CAD build for the part. Positions are in the model's coordinates, mm. Round coordinates to 2 decimals unless told otherwise and drop trailing zeros. Loops run counter-clockwise (first coordinate to the right, second up) from the corner with the lowest first, then second, coordinate; pieces in that order, holes last. Notation, with made-up numbers: (-20, 16.5) - (22, 16.5) arc R24 ccw to (22, 47.5) - close; hole circle Ø3 at (-16, 88). An arc over 180 degrees is marked (long way). One line per question, with ' | ' between items.
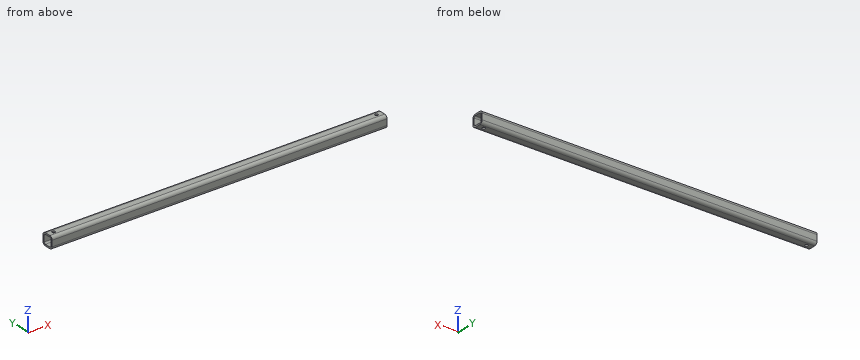
```python
from build123d import *

# Parameters (mm, degrees)
STRUCTURAL_MEMBER1_DEPTH = 1422.4
SKETCH12_R               = 6.35
CUT_EXTRUDE1_DEPTH       = 744.764894646


with BuildPart() as part:
    # Sketch11 → Structural Member1 (new body)
    with BuildSketch(Plane.YZ.offset(-741.593162393)):
        with BuildLine():
            Line((-12.7, -25.4), (12.7, -25.4))
            ThreePointArc((12.7, -25.4), (21.680256121, -21.680256121), (25.4, -12.7))
            Line((25.4, -12.7), (25.4, 12.7))
            ThreePointArc((25.4, 12.7), (21.680256121, 21.680256121), (12.7, 25.4))
            Line((12.7, 25.4), (-12.7, 25.4))
            ThreePointArc((-12.7, 25.4), (-21.680256121, 21.680256121), (-25.4, 12.7))
            Line((-25.4, 12.7), (-25.4, -12.7))
            ThreePointArc((-25.4, -12.7), (-21.680256121, -21.680256121), (-12.7, -25.4))
        make_face()
        with BuildLine():
            Line((-12.7, -19.05), (12.7, -19.05))
            ThreePointArc((12.7, -19.05), (17.190128061, -17.190128061), (19.05, -12.7))
            Line((19.05, -12.7), (19.05, 12.7))
            ThreePointArc((19.05, 12.7), (17.190128061, 17.190128061), (12.7, 19.05))
            Line((12.7, 19.05), (-12.7, 19.05))
            ThreePointArc((-12.7, 19.05), (-17.190128061, 17.190128061), (-19.05, 12.7))
            Line((-19.05, 12.7), (-19.05, -12.7))
            ThreePointArc((-19.05, -12.7), (-17.190128061, -17.190128061), (-12.7, -19.05))
        make_face(mode=Mode.SUBTRACT)
    extrude(amount=STRUCTURAL_MEMBER1_DEPTH)

    # Sketch12 → Cut-Extrude1 (cut, through all)
    with BuildSketch(Plane.XY.offset(25.4)):
        with Locations((-716.193162393, 0)):
            Circle(SKETCH12_R)
        with Locations((655.406837607, 0)):
            Circle(SKETCH12_R)
    extrude(amount=-CUT_EXTRUDE1_DEPTH, mode=Mode.SUBTRACT)


solid = part.part
```
(1) Cut at B-B, the plane x = 386. Write the cut outline in (y, z), then the cut area to 3 significant figures.
Results found:
outline: (-25.4, -12.7) arc R12.7 ccw to (-12.7, -25.4) - (12.7, -25.4) arc R12.7 ccw to (25.4, -12.7) - (25.4, 12.7) arc R12.7 ccw to (12.7, 25.4) - (-12.7, 25.4) arc R12.7 ccw to (-25.4, 12.7) - close; hole (-19.05, -12.7) arc R6.35 ccw to (-12.7, -19.05) - (12.7, -19.05) arc R6.35 ccw to (19.05, -12.7) - (19.05, 12.7) arc R6.35 ccw to (12.7, 19.05) - (-12.7, 19.05) arc R6.35 ccw to (-19.05, 12.7) - close | area: 1,030 mm²
(2) Cut at A-A, the plane z = 0.5. Write the cut outline in (x, y), then the cut area to 3 significant figures.
Results found:
outline: (-741.59, -25.4) - (680.81, -25.4) - (680.81, -19.05) - (-741.59, -19.05) - close; (-741.59, 19.05) - (680.81, 19.05) - (680.81, 25.4) - (-741.59, 25.4) - close | area: 18,100 mm²
(3) Drop flat-ended pins along their axis: P1, Ø5, axis at x = -559, z = 18, coming from the +Y side; P2, Ø2, axis at x = -270, y = 14, coming from the +Z side. Give the stop position or say it passes through.
Results found:
P1: stops at y = 25.09 | P2: stops at z = 25.4
(4) Probe L1, parallel to Y at x = -501, z = -5; L2, parallel to Z at x = 69.5, y = -13; L3, parallel to X at y = 4, z = -22. List the from-to ranges inside material, lowest first.
Results found:
L1: y = -25.4 to -19.05, 19.05 to 25.4 | L2: z = -25.4 to -19.04, 19.04 to 25.4 | L3: x = -741.59 to -721.12, -711.26 to 650.48, 660.34 to 680.81
